Input: part model. Units: mm. Frame: model coordinates. Face numbers are marked on the shaded views. A direction names the side the tool comes from. Round coordinates to 2 decimals unless told otherwise and drop trailing zeros. Loops run counter-clockwise (first coordinate to the right, second up) from the corner with the lowest first, then second, coordinate; pieces in that order, holes last. Notation, with made-up numbers: (81.5, -12.75) -> (115.5, -12.75) arc R11 ccw to (115.5, -7.75) -> close; hole circle Ø5 at (-13.5, 79.25). An arc over 180 degrees is marked (long way). Answer in a Markdown table with one row per item. Add a question column.
Q1. Section D-D, the plane z = 1.5. Output: boundary loops of the cut face in (x, y), and give its area (3 significant figures).
Q2. Pin query (flat end, axial travel): pin 1 (5 mm diameter, centred on x = 1, y = 46.5, fed in from -Z); pin 2 (1.8 mm diameter, centred on y = 30, z = -6.5, fed in from +X); pin 3 (23.5 mm diameter, centred on x = -7, y = 26, fed in from +Z); pin 4 (6.5 mm diameter, centred on y = 31.5, z = -7, fed in from -X). Return the tip coordinate at first contact, or that it passes through.
Q3. Section A-A, the plane x = 32.5. Output: boundary loops of the cut face in (y, z), and give its area (3 significant figures).
Q4. Section B-B, the plane z = -18. Output: boundary loops of the cut face in (x, y).
Q5. Section C-C, the plane x = -9. Output: boundary loops of the cut face in (y, z), and give its area (3 significant figures).
Q6. Reachability of the marked faces 1, 2 and 3 from +Z, -Z, +X, -X, +Y, -Y: full face, straight path, thin tool, end or side. Return the list, or none.
Q7. Mould query, pull axis X, two halves, no side actions, for the marked faces 4 and 5. Classes: pulls with the +X half, pulls with the -X half, needs draft (parallel to the pull), parting line crosses it, or undercut.
Q8. Ray query, L1, parallel to Z at x = -42, y = 38.5; L2, parallel to Y at x = -10, z = 2; L3, parallel to Z at x = 0.5, y = 39. Return the intervals inside material, ascending. Write a range as from..to.
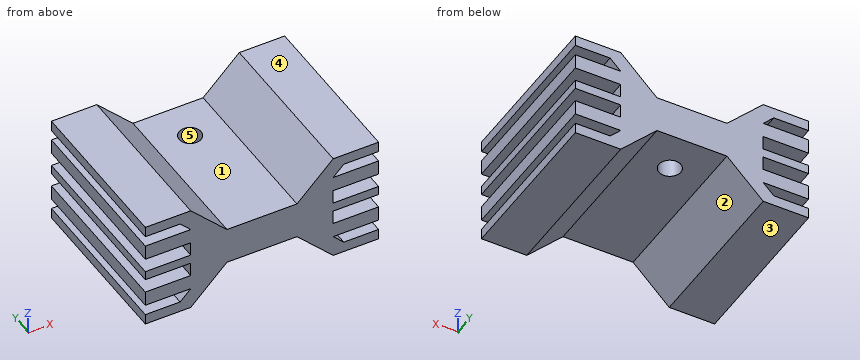
```python
from build123d import *

# Parameters (mm, degrees)
BOSS_EXTRUDE1_DEPTH = 70
SKETCH3_R           = 4.630574493
CUT_EXTRUDE1_DEPTH  = 97.893202961


with BuildPart() as part:
    # Sketch1 → Boss-Extrude1 (new body)
    with BuildSketch(Plane(origin=(0, 0, 0), x_dir=(1, 0, 0), z_dir=(0, 1, 0))):
        Polygon((-59.338025707, 25.167507455), (-40.104320822, 25.167507455), (-24.758279691, 9.821466324), (4.910733162, 9.821466324), (20.256774293, 25.167507455), (39.490479177, 25.167507455), (39.490479177, 20.666002056), (24.758279691, 20.666002056), (20.256774293, 16.164496658), (39.490479177, 16.164496658), (39.490479177, 9.821466324), (20.256774293, 9.821466324), (20.256774293, 3.887663753), (39.490479177, 3.887663753), (39.490479177, 0), (20.256774293, 0), (20.256774293, -5.933802571), (39.490479177, -5.933802571), (39.490479177, -12.276832905), (20.256774293, -12.276832905), (24.758279691, -16.778338303), (39.490479177, -16.778338303), (39.490479177, -21.279843702), (20.256774293, -21.279843702), (4.910733162, -5.933802571), (-24.758279691, -5.933802571), (-40.104320822, -21.279843702), (-59.338025707, -21.279843702), (-59.338025707, -16.778338303), (-44.605826221, -16.778338303), (-40.104320822, -12.276832905), (-59.338025707, -12.276832905), (-59.338025707, -5.933802571), (-40.104320822, -5.933802571), (-40.104320822, 0), (-59.338025707, 0), (-59.338025707, 3.887663753), (-40.104320822, 3.887663753), (-40.104320822, 9.821466324), (-59.338025707, 9.821466324), (-59.338025707, 16.164496658), (-40.104320822, 16.164496658), (-44.605826221, 20.666002056), (-59.338025707, 20.666002056), align=None)
    extrude(amount=BOSS_EXTRUDE1_DEPTH)

    # Sketch3 → Cut-Extrude1 (cut, through all)
    with BuildSketch(Plane(origin=(0, 0, -9.821466324), x_dir=(-1, 0, 0), z_dir=(0, 0, -1))):
        with Locations((9.923773265, 53.534976089)):
            Circle(SKETCH3_R)
    extrude(amount=-CUT_EXTRUDE1_DEPTH, mode=Mode.SUBTRACT)


solid = part.part
```
Answer block:
| question | item | result |
|---|---|---|
| 1 | outline | (-40.1, 0) -> (20.26, 0) -> (20.26, 70) -> (-40.1, 70) -> close; hole circle Ø9.26 at (-9.92, 53.53) |
| 1 | area | 4,160 mm^2 |
| 2 | pin 1 | z = -9.82 |
| 2 | pin 2 | x = 20.26 |
| 2 | pin 3 | z = 5.93 |
| 2 | pin 4 | x = -59.34 |
| 3 | outline | (0, -25.17) -> (70, -25.17) -> (70, -20.67) -> (0, -20.67) -> close; (0, -16.16) -> (70, -16.16) -> (70, -9.82) -> (0, -9.82) -> close; (0, -3.89) -> (70, -3.89) -> (70, 0) -> (0, 0) -> close; (0, 5.93) -> (70, 5.93) -> (70, 12.28) -> (0, 12.28) -> close; (0, 16.78) -> (70, 16.78) -> (70, 21.28) -> (0, 21.28) -> close |
| 3 | area | 1,790 mm^2 |
| 4 | outline | (-41.94, 0) -> (-32.94, 0) -> (-32.94, 70) -> (-41.94, 70) -> close; (13.09, 0) -> (22.09, 0) -> (22.09, 70) -> (13.09, 70) -> close |
| 5 | outline | (0, -9.82) -> (49, -9.82) -> (49, 5.93) -> (0, 5.93) -> close; (58.07, -9.82) -> (70, -9.82) -> (70, 5.93) -> (58.07, 5.93) -> close |
| 5 | area | 960 mm^2 |
| 6 | face 1 | +Z, +Y, -Y |
| 6 | face 2 | -Z, +Y, -Y |
| 6 | face 3 | -Z, +X, -X, +Y, -Y |
| 7 | face 4 | needs draft |
| 7 | face 5 | undercut |
| 8 | L1 | -25.17..-18.06, -16.16..-9.82, -3.89..0, 5.93..12.28, 14.17..21.28 |
| 8 | L2 | 0..48.91, 58.16..70 |
| 8 | L3 | -9.82..5.93 |
